Check sheet for the modelled part. Datum: model origin and axes. Units: mm. Round coordinates to 2 decimals unless told otherwise and drop trailing zeros. Write each loop counter-clockwise with the first axis right and the second up, starting at its lowest first coordinate (ties: lowest second). Pieces come first, ordered by that corner, then holes. Notation, with made-up numbers: M 24.5,48 L 39.5,48 A15 cw 39.5,60 Z; hole C 54,-26.5 d6. An arc over 180 degrees is marked long. Put each result on its own line as item: value.
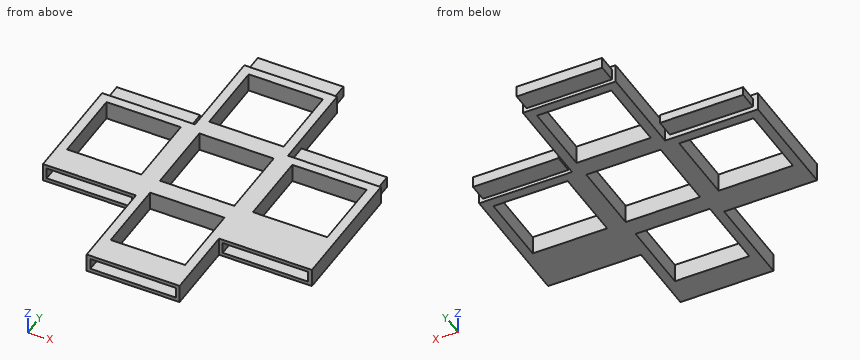
```python
from build123d import *

# Parameters (mm, degrees)
F0_W      = 127
F0_H      = 127
F0_W_2    = 101.6
F0_H_2    = 101.6
F1_DEPTH  = 25.4
F2_W      = 116.84
F2_H      = 15.24
F3_DEPTH  = 25.4
F5_W      = 113.6791649616
F5_H      = 12.0791649616
F6_DEPTH  = 25.4
F7_W      = 5.08
F7_H      = 15.24
F7_W_2    = 111.76
F8_DEPTH  = 25.4
F9_W      = 127
F9_H      = 25.4
F9_W_2    = 116.84
F9_H_2    = 15.24
F10_DEPTH = 25.4
F11_W     = 127
F11_H     = 25.4
F11_W_2   = 116.84
F11_H_2   = 15.24
F12_DEPTH = 25.4
F13_W     = 127
F13_H     = 25.4
F13_W_2   = 116.84
F13_H_2   = 15.24
F14_DEPTH = 25.4
F15_W     = 127
F15_H     = 25.4
F15_W_2   = 116.84
F15_H_2   = 15.24
F16_DEPTH = 25.4


with BuildPart() as f1:
    # F0 (on Top) → F1 (new body)
    with BuildSketch(Plane.XY):
        with Locations((-0.1885456222, 127.423350506)):
            Rectangle(F0_W, F0_H)
        with Locations((-0.1885456222, 127.423350506)):
            Rectangle(F0_W_2, F0_H_2, mode=Mode.SUBTRACT)
        with Locations((-0.1885456222, 0.423350506)):
            Rectangle(F0_W, F0_H)
        with Locations((-0.1885456222, 0.423350506)):
            Rectangle(F0_W_2, F0_H_2, mode=Mode.SUBTRACT)
        with Locations((-127.1885456222, 0.423350506)):
            Rectangle(F0_W, F0_H)
        with Locations((-127.1885456222, 0.423350506)):
            Rectangle(F0_W_2, F0_H_2, mode=Mode.SUBTRACT)
        with Locations((126.8114543778, 0.423350506)):
            Rectangle(F0_W, F0_H)
        with Locations((126.8114543778, 0.423350506)):
            Rectangle(F0_W_2, F0_H_2, mode=Mode.SUBTRACT)
        with Locations((-0.1885456222, -126.576649494)):
            Rectangle(F0_W, F0_H)
        with Locations((-0.1885456222, -126.576649494)):
            Rectangle(F0_W_2, F0_H_2, mode=Mode.SUBTRACT)
    extrude(amount=F1_DEPTH)

    # F2 (on face) → F3 (join)
    with BuildSketch(Plane(origin=(0, 190.923350506, 0), x_dir=(-1, 0, 0), z_dir=(0, 1, 0))):
        with Locations((0.1885456222, 12.7)):
            Rectangle(F2_W, F2_H)
    extrude(amount=F3_DEPTH)

    # F5 (on face) → F6 (join)
    with BuildSketch(Plane(origin=(0, 63.923350506, 0), x_dir=(-1, 0, 0), z_dir=(0, 1, 0))):
        with Locations((127.1885456222, 12.7)):
            Rectangle(F5_W, F5_H)
    extrude(amount=F6_DEPTH)

    # F7 (on face) → F8 (join)
    with BuildSketch(Plane(origin=(0, 63.923350506, 0), x_dir=(-1, 0, 0), z_dir=(0, 1, 0))):
        with Locations((-182.6914543778, 12.7)):
            Rectangle(F7_W, F7_H)
        with Locations((-124.2714543778, 12.7)):
            Rectangle(F7_W_2, F7_H)
    extrude(amount=F8_DEPTH)

    # F9 (on face) → F10 (join)
    with BuildSketch(Plane.XZ.offset(63.076649494)):
        with Locations((126.8114543778, 12.7)):
            Rectangle(F9_W, F9_H)
        with Locations((126.8114543778, 12.7)):
            Rectangle(F9_W_2, F9_H_2, mode=Mode.SUBTRACT)
        with Locations((126.8114543778, 12.7)):
            Rectangle(F9_W_2, F9_H_2)
    extrude(amount=F10_DEPTH)

    # F11 (on face) → F12 (join)
    with BuildSketch(Plane.XZ.offset(88.476649494)):
        with Locations((126.8114543778, 12.7)):
            Rectangle(F11_W, F11_H)
        with Locations((126.8114543778, 12.7)):
            Rectangle(F11_W_2, F11_H_2, mode=Mode.SUBTRACT)
    extrude(amount=F12_DEPTH)

    # F13 (on face) → F14 (join)
    with BuildSketch(Plane.XZ.offset(190.076649494)):
        with Locations((-0.1885456222, 12.7)):
            Rectangle(F13_W, F13_H)
        with Locations((-0.1885456222, 12.7)):
            Rectangle(F13_W_2, F13_H_2, mode=Mode.SUBTRACT)
    extrude(amount=F14_DEPTH)

    # F15 (on face) → F16 (join)
    with BuildSketch(Plane.XZ.offset(63.076649494)):
        with Locations((-127.1885456222, 12.7)):
            Rectangle(F15_W, F15_H)
        with Locations((-127.1885456222, 12.7)):
            Rectangle(F15_W_2, F15_H_2, mode=Mode.SUBTRACT)
    extrude(amount=F16_DEPTH)


solid = f1.part
```
1. Cross-section at C-C (x = 7). Enter the section's corners in (y, z), then the cut area to 3 significant figures.
Computed values:
outline: M -215.48,0 L -177.38,0 L -177.38,25.4 L -215.48,25.4 L -215.48,20.32 L -190.08,20.32 L -190.08,5.08 L -215.48,5.08 Z; M -75.78,0 L -50.38,0 L -50.38,25.4 L -75.78,25.4 Z; M 51.22,0 L 76.62,0 L 76.62,25.4 L 51.22,25.4 Z; M 178.22,0 L 190.92,0 L 190.92,5.08 L 216.32,5.08 L 216.32,20.32 L 190.92,20.32 L 190.92,25.4 L 178.22,25.4 Z
area: 2,580 mm2
2. Cross-section at D-D (z = 13.5). Count the separate pieces of the cut face and the enclosed holes in it, then the cut area to 3 significant figures.
Computed values:
separate pieces: 1
enclosed holes: 5
area: 41,900 mm2
3. Cross-section at B-B (x = 164.5). Enter the section's corners in (y, z), then the cut area to 3 significant figures.
Computed values:
outline: M -113.88,0 L -50.38,0 L -50.38,25.4 L -113.88,25.4 L -113.88,20.32 L -88.48,20.32 L -88.48,5.08 L -113.88,5.08 Z; M 51.22,0 L 63.92,0 L 63.92,5.08 L 89.32,5.08 L 89.32,20.32 L 63.92,20.32 L 63.92,25.4 L 51.22,25.4 Z
area: 1,940 mm2
4. Scan lines: probe 1 along Y at (x, z) = (43.5, 6.5); probe 2 along X at (y, z) = (43, 24.25); probe 3 along Y at (x, z) = (45, 22). Record each from-to range of solid material in increasing order.
Computed values:
probe 1: y = -190.08 to -177.38, -75.78 to -50.38, 51.22 to 76.62, 178.22 to 216.32
probe 2: x = -190.69 to -177.99, -76.39 to -50.99, 50.61 to 76.01, 177.61 to 190.31
probe 3: y = -215.48 to -177.38, -75.78 to -50.38, 51.22 to 76.62, 178.22 to 190.92
5. Depth check by flat-ended pin: pin 1 Ø3 at (y, z) = (-150, 4) entering from -X; pin 2 Ø4.5 at (x, z) = (111.5, 12) entering from +Y; pin 3 Ø12.5 at (x, z) = (15, 12.5) entering from -Y; pin 4 Ø7.5 at (x, z) = (-18.5, 8) entering from -Y. Enter the tip coordinate at first touch or a pass-through.
Computed values:
pin 1: stops at x = -63.69
pin 2: stops at y = 89.32
pin 3: stops at y = -190.08
pin 4: stops at y = -215.48
6. Cross-section at A-A (y = 149). Enter the section's corners in (x, z), then the cut area to 3 significant figures.
Computed values:
outline: M -63.69,0 L -50.99,0 L -50.99,25.4 L -63.69,25.4 Z; M 50.61,0 L 63.31,0 L 63.31,25.4 L 50.61,25.4 Z
area: 645 mm2
